Could you check a few things on this drawing? It's one solid part, dimensions in mm from its lowest x, y, z. A direction names the side the tool comes from. Give positions to 0.01 mm unless a question says otherwise; leave off trailing zeros. Loops run counter-clockwise (first coordinate to the right, second up) from the corner with the lowest first, then second, coordinate; pieces in that order, holes last.
Q1. Suppose I cut it at C-C (x = 1). List the corners of the cut face in (y, z) for me, and give its area (3 significant figures).
Q2. I'm going to push flat-ended pins straight in: P1, Ø3, axis at y = 3, z = 1, coming from the -X side; P2, Ø1.5, axis at x = 1.5, y = 2.5, coming from the -Z side; P3, Ø1.5, axis at y = 4.5, z = 3, coming from the +X side (3 decimals). Where does each tip first touch, or does it pass through?
Q3. Suppose I cut it at B-B (z = 4.6). List the corners of the cut face in (x, y) for me.
Q4. Suppose I cut it at A-A (y = 2). List the corners of the cut face in (x, z) for me, and give its area (3 significant figures).
Q5. I need wall thicknesses on probe 1 along X at (y, z) = (1.5, 2.75); probe 2 along X at (y, z) = (2.85, 4.75). Which ranges of each line are inside material? Lowest first, please.
Q6. For the marked faces 1 and 2, which set-ups out of +Z, -Z, +X, -X, +Y, -Y let a thin tool reach every point of the face, with its end or its side?
Q7. Suppose I cut it at D-D (y = 4.6). List the corners of the cut face in (x, z) for me, and give its area (3 significant figures).
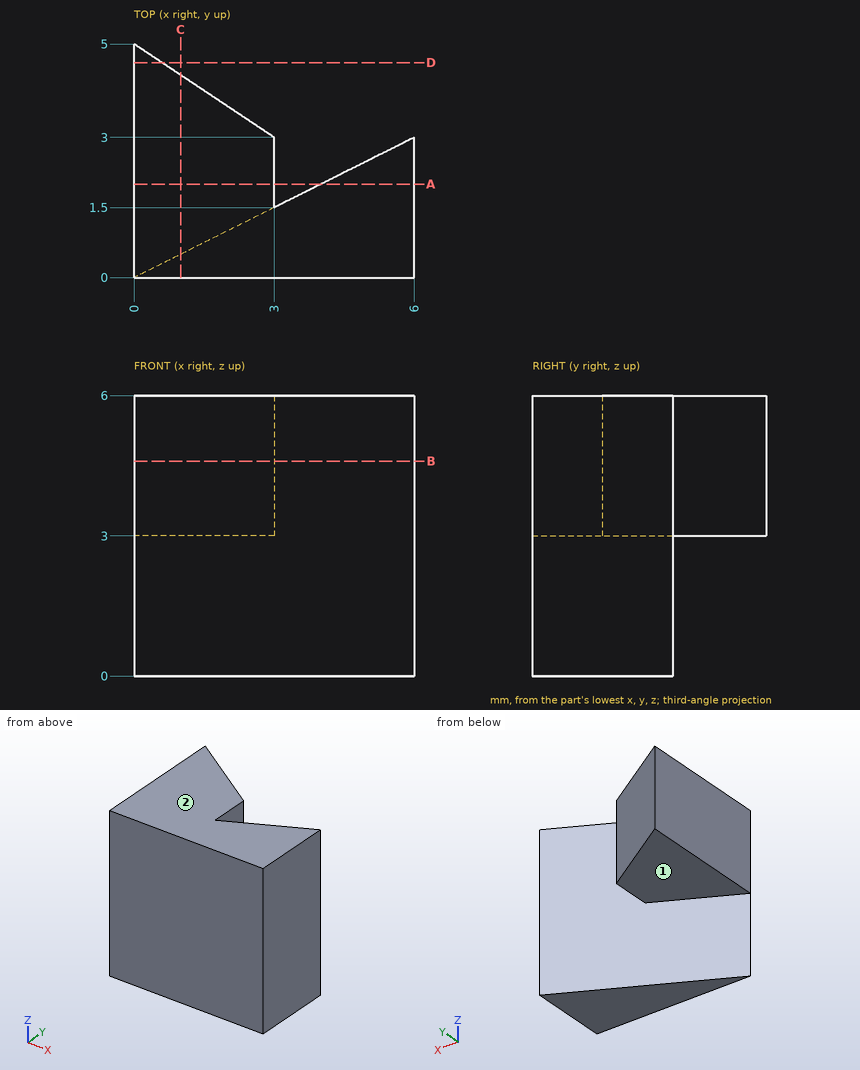
Solutions:
1. outline: (0, 0) - (0.5, 0) - (0.5, 3) - (4.33, 3) - (4.33, 6) - (0, 6) - close
1. area: 14.5 mm2
2. P1: stops at x = 3
2. P2: stops at z = 3
2. P3: stops at x = 1.875
3. outline: (0, 0) - (6, 0) - (6, 3) - (3, 1.5) - (3, 3) - (0, 5) - close
4. outline: (0, 3) - (3, 3) - (3, 6) - (0, 6) - close; (4, 0) - (6, 0) - (6, 6) - (4, 6) - close
4. area: 21.0 mm2
5. probe 1: x = 3 to 6
5. probe 2: x = 0 to 3, 5.7 to 6
6. face 1: -Z, -X, +Y
6. face 2: +Z, +X, -X, +Y, -Y
7. outline: (0, 3) - (0.6, 3) - (0.6, 6) - (0, 6) - close
7. area: 1.80 mm2
